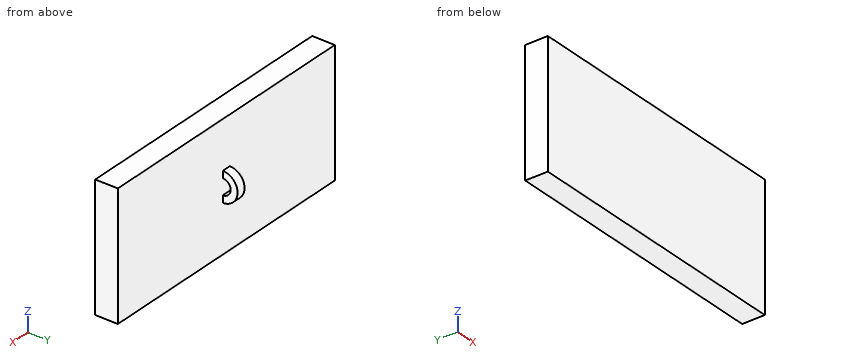
```python
from build123d import *

# Parameters (mm, degrees)
SKETCH2_W           = 123.909820238
SKETCH2_H           = 55.24312819
BOSS_EXTRUDE2_DEPTH = 10
SKETCH3_W           = 4
SKETCH3_H           = 3.05525832
REVOLVE4_ANGLE      = 180


with BuildPart() as part:
    # Sketch2 → Boss-Extrude2 (new body)
    with BuildSketch(Plane(origin=(0, 0, 0), x_dir=(1, 0, 0), z_dir=(0, 1, 0))):
        Rectangle(SKETCH2_W, SKETCH2_H)
    extrude(amount=BOSS_EXTRUDE2_DEPTH)

    # Sketch3 → Revolve4 (revolve)
    with BuildSketch(Plane(origin=(0, 10, 0), x_dir=(1, 0, 0), z_dir=(0, 1, 0))):
        with Locations((0, 4.999513614)):
            Rectangle(SKETCH3_W, SKETCH3_H)
    revolve(axis=Axis((-61.954910119, 10, 0), (1, 0, 0)), revolution_arc=REVOLVE4_ANGLE)


solid = part.part
```
Verification items for the finished model (mm, model axes). Give positions to 0.01 mm unless a question says otherwise; leave off trailing zeros. Order: outer loops, then holes, each group sorted by start corner. A loop starts at its lowest first (then second) coordinate and runs counter-clockwise, first axis right, second up. Notation, with made-up numbers: M 61.5,43 L 89.5,43 A28 cw 89.5,77 Z; hole C -35,56 d9. An arc over 180 degrees is marked long. Answer in a Markdown table with one row per item. Add a question column.
Item 1: Section check C-C, the plane x = -43. Enter the section's corners in (y, z), and give its area (3 significant figures).
Item 2: Gauge pin test, flat ends, axial feed: pin 1 (6 mm diameter, centred on x = -10, y = 10.5, fed in from -Z); pin 2 (7 mm diameter, centred on y = 14.5, z = -0.5, fed in from +X); pin 3 (5 mm diameter, centred on y = 13, z = -3, fed in from -X); pin 4 (16.5 mm diameter, centred on x = 11, z = -4.5, fed in from +Y). Record the tip position at first contact, or that the pin passes through.
Item 3: Section check B-B, the plane y = 11.5. Enter the section's corners in (x, z), and give its area (3 significant figures).
Item 4: Section check A-A, the plane z = 0. Enter the section's corners in (x, y).
Item 5: Section check D-D, the plane z = 23. Enter the section's corners in (x, y), and give its area (3 significant figures).
Item 6: Scan lines: probe 1 along X at (y, z) = (13.75, -4); probe 2 along Y at (x, z) = (31.5, -21.5); probe 3 along Z at (x, y) = (0, 10.75). Record each from-to range of solid material in increasing order. Write a range as from..to.
Filled sheet:
| question | item | result |
|---|---|---|
| 1 | outline | M 0,-27.62 L 10,-27.62 L 10,27.62 L 0,27.62 Z |
| 1 | area | 552 mm^2 |
| 2 | pin 1 | stops at z = -27.62 |
| 2 | pin 2 | stops at x = 2 |
| 2 | pin 3 | stops at x = -2 |
| 2 | pin 4 | stops at y = 10 |
| 3 | outline | M -2,-6.35 L 2,-6.35 L 2,-3.13 L -2,-3.13 Z; M -2,3.13 L 2,3.13 L 2,6.35 L -2,6.35 Z |
| 3 | area | 25.8 mm^2 |
| 4 | outline | M -61.95,0 L 61.95,0 L 61.95,10 L -61.95,10 Z; M -2,13.47 L 2,13.47 L 2,16.53 L -2,16.53 Z |
| 5 | outline | M -61.95,0 L 61.95,0 L 61.95,10 L -61.95,10 Z |
| 5 | area | 1,240 mm^2 |
| 6 | probe 1 | x = -2..2 |
| 6 | probe 2 | y = 0..10 |
| 6 | probe 3 | z = -6.48..-3.39, 3.39..6.48 |
